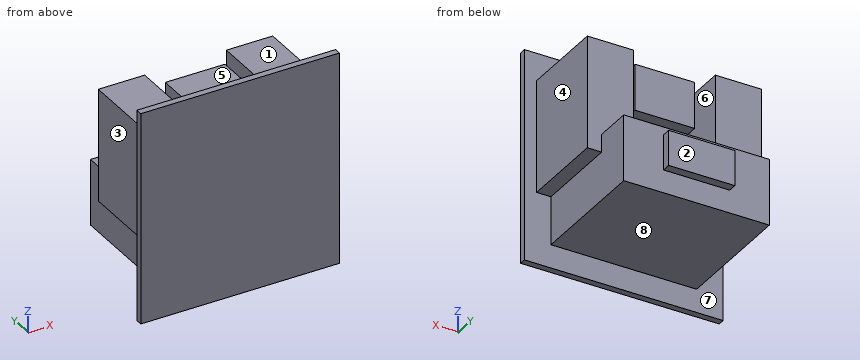
```python
from build123d import *

# Parameters (mm, degrees)
SKETCH_1_W      = 450
SKETCH_1_H      = 480
EXTRUDE_1_DEPTH = 15
SKETCH_2_W      = 330
SKETCH_2_H      = 150
EXTRUDE_2_DEPTH = 280
SKETCH_3_W      = 105
SKETCH_3_H      = 255
EXTRUDE_3_DEPTH = 195
SKETCH_4_W      = 105
SKETCH_4_H      = 255
EXTRUDE_4_DEPTH = 195
SKETCH_5_W      = 135
SKETCH_5_H      = 105
EXTRUDE_5_DEPTH = 158
SKETCH_6_W      = 150
SKETCH_6_H      = 80
EXTRUDE_6_DEPTH = 300


with BuildPart() as part:
    # 草图1 → 凸台-拉伸1 (new body)
    with BuildSketch(Plane(origin=(0, 0, 0), x_dir=(1, 0, 0), z_dir=(0, 1, 0))):
        Rectangle(SKETCH_1_W, SKETCH_1_H)
    extrude(amount=-EXTRUDE_1_DEPTH)

    # 草图2 → 凸台-拉伸2 (add)
    with BuildSketch(Plane(origin=(0, 0, 0), x_dir=(1, 0, 0), z_dir=(0, 1, 0))):
        with Locations((0, 112)):
            Rectangle(SKETCH_2_W, SKETCH_2_H)
    extrude(amount=EXTRUDE_2_DEPTH)

    # 草图3 → 凸台-拉伸3 (add)
    with BuildSketch(Plane(origin=(0, 0, 0), x_dir=(1, 0, 0), z_dir=(0, 1, 0))):
        with Locations((-145, -50)):
            Rectangle(SKETCH_3_W, SKETCH_3_H)
    extrude(amount=EXTRUDE_3_DEPTH)

    # 草图4 → 凸台-拉伸4 (add)
    with BuildSketch(Plane(origin=(0, 0, 0), x_dir=(1, 0, 0), z_dir=(0, 1, 0))):
        with Locations((145, -50)):
            Rectangle(SKETCH_4_W, SKETCH_4_H)
    extrude(amount=EXTRUDE_4_DEPTH)

    # 草图5 → 凸台-拉伸5 (add)
    with BuildSketch(Plane(origin=(0, 0, 0), x_dir=(1, 0, 0), z_dir=(0, 1, 0))):
        with Locations((0, -120)):
            Rectangle(SKETCH_5_W, SKETCH_5_H)
    extrude(amount=EXTRUDE_5_DEPTH)

    # 草图6 → 凸台-拉伸6 (add)
    with BuildSketch(Plane(origin=(0, 0, 0), x_dir=(1, 0, 0), z_dir=(0, 1, 0))):
        with Locations((0, 95)):
            Rectangle(SKETCH_6_W, SKETCH_6_H)
    extrude(amount=EXTRUDE_6_DEPTH)


solid = part.part
```
For this review, take the finished solid that the model builds, in its own axes (mm). Face numbers are marked on the shaded views. A direction names the side the tool comes from. Round coordinates to 2 decimals unless told otherwise and drop trailing zeros. Write each loop counter-clockwise with the first axis right and the second up, starting at its lowest first coordinate (ties: lowest second). Pieces come first, ordered by that corner, then holes. Notation, with made-up numbers: (17, 12.25) - (47, 12.25) arc R26 ccw to (47, 35.25) - close; hole circle Ø5 at (-31.5, 2). An arc over 180 degrees is marked (long way). Answer as CSV lines item,"result". Start each with the question number.
(1) Add section D-D, the plane x = 133. State the section outline as (y, z) points, plus the area to 3 significant figures.
(2) Machinability: for the marked faces 1, 2, 3, 4 and 5, which of the approach directions +Z, -Z, +X, -X, +Y, -Y give a long, thin tool a straight path to every point of the face, cutting with its end or side? Answer none if there is none.
(3) Add section A-A, the plane y = 119.5. State the section outline as (x, z) points, plus the area to 3 significant figures.
(4) Mouldability with a two-part tool opening along Z and no side actions: class the marked faces 6, 7 and 8 as +Z half, -Z half, draft (parallel to the pull), parting line (faces both ways), or undercut.
(5) Add section C-C, the plane x = 6. State the section outline as (y, z) points.
(6) For line 1 (X direction, y = 116.5, z = 138.5); line 2 (X direction, y = 148.5, z = -28); line 3 (Z direction, x = 40.5, y = 29), list the stretches that pass through material, from the lowest coordinate up.
(7) For pin 1 (6 mm diameter, centred on x = 19.5, y = 134, fed in from +Z); pin 2 (2 mm diameter, centred on x = -128.5, z = 82, fed in from +Y); pin 3 (2 mm diameter, centred on y = 236, z = -145, fed in from -X), all flat-tipped, find the tip position at first contact; note any pin that passes through.
(8) Add section B-B, the plane z = 44.5. State the section outline as (x, y) points, plus the area to 3 significant figures.
From the geometry:
1,outline,"(-15, -240) - (0, -240) - (0, -187) - (280, -187) - (280, -37) - (195, -37) - (195, 177.5) - (0, 177.5) - (0, 240) - (-15, 240) - close"
1,area,"91,000 mm²"
2,face 1,"+Z, +X, -X, +Y"
2,face 2,"+Z, -Z, +X, -X, +Y"
2,face 3,"+Z, -Z, -X, +Y"
2,face 4,"+Z, -Z, +X, +Y"
2,face 5,"+Z, +Y"
3,outline,"(-197.5, -77.5) - (-165, -77.5) - (-165, -187) - (165, -187) - (165, -77.5) - (197.5, -77.5) - (197.5, 177.5) - (92.5, 177.5) - (92.5, -37) - (-92.5, -37) - (-92.5, 177.5) - (-197.5, 177.5) - close; (-67.5, 67.5) - (67.5, 67.5) - (67.5, 172.5) - (-67.5, 172.5) - close"
3,area,"111,000 mm²"
4,face 6,"draft"
4,face 7,"undercut"
4,face 8,"-Z half"
5,outline,"(-15, -240) - (0, -240) - (0, -187) - (280, -187) - (280, -135) - (300, -135) - (300, -55) - (280, -55) - (280, -37) - (0, -37) - (0, 67.5) - (158, 67.5) - (158, 172.5) - (0, 172.5) - (0, 240) - (-15, 240) - close"
6,line 1,"x = -197.5 to -92.5, -67.5 to 67.5, 92.5 to 197.5"
6,line 2,"x = -197.5 to -92.5, 92.5 to 197.5"
6,line 3,"z = -187 to -37, 67.5 to 172.5"
7,pin 1,"stops at z = 172.5"
7,pin 2,"stops at y = 195"
7,pin 3,"stops at x = -165"
8,outline,"(-225, -15) - (225, -15) - (225, 0) - (197.5, 0) - (197.5, 195) - (92.5, 195) - (92.5, 0) - (-92.5, 0) - (-92.5, 195) - (-197.5, 195) - (-197.5, 0) - (-225, 0) - close"
8,area,"47,700 mm²"
